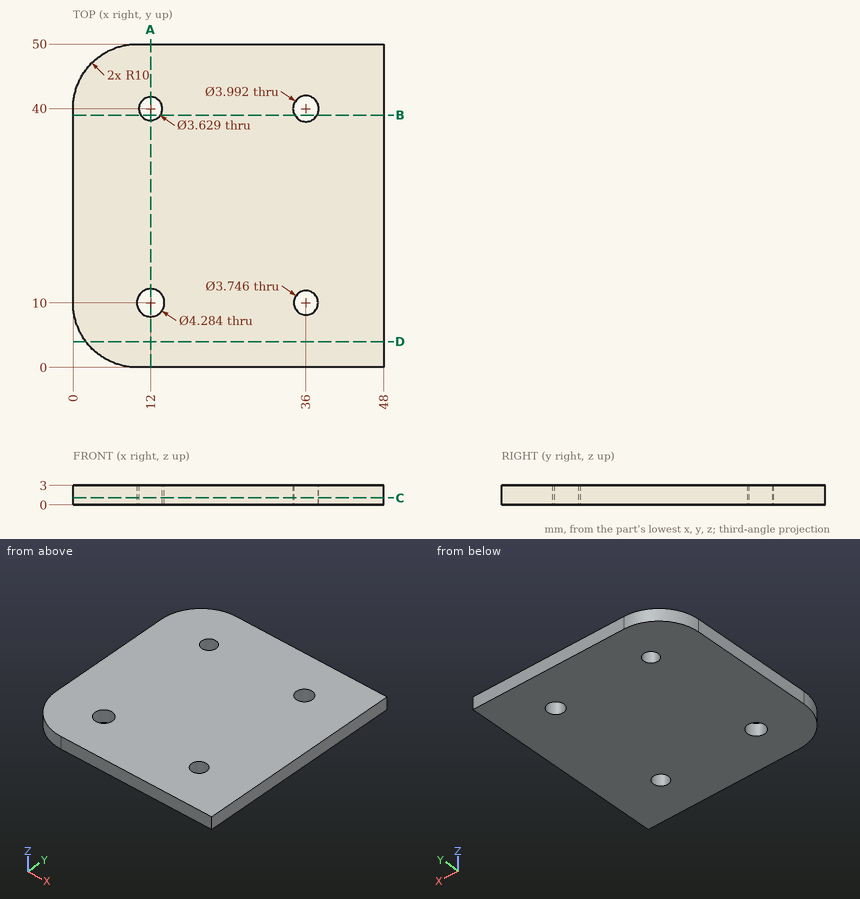
Can you work these out from the drawing? Everything is in mm from the part's minimum corner. Give positions to 0.01 mm unless a question says otherwise; leave off trailing zeros. Order: outer loops, then holes, each group sorted by start corner. A loop starts at its lowest first (then second) coordinate and runs counter-clockwise, first axis right, second up.
1. Suppose I cut it at A-A (x = 12). List the corners of the cut face in (y, z) for me (1 decimal).
2. Suppose I cut it at D-D (y = 4). List the corners of the cut face in (x, z) for me.
3. Suppose I cut it at B-B (y = 39). List the corners of the cut face in (x, z) for me.
4. Suppose I cut it at C-C (z = 1.1). List the corners of the cut face in (x, y) for me (1 decimal), plus the area to 3 significant figures.
5. I need wall thicknesses on L1, parallel to Y at x = 36, z = 1.75 (1 decimal); L2, parallel to Y at x = 36.5, z = 1.15 (1 decimal); L3, parallel to X at y = 39.5, z = 0.8 (1 decimal). Which ranges of each line are inside material? Lowest first, please.
Solved:
1. outline: (0, 0) - (7.9, 0) - (7.9, 3) - (0, 3) - close; (12.1, 0) - (38.2, 0) - (38.2, 3) - (12.1, 3) - close; (41.8, 0) - (50, 0) - (50, 3) - (41.8, 3) - close
2. outline: (2, 0) - (48, 0) - (48, 3) - (2, 3) - close
3. outline: (0, 0) - (10.49, 0) - (10.49, 3) - (0, 3) - close; (13.51, 0) - (34.27, 0) - (34.27, 3) - (13.51, 3) - close; (37.73, 0) - (48, 0) - (48, 3) - (37.73, 3) - close
4. outline: (0, 10) arc R10 ccw to (10, 0) - (48, 0) - (48, 50) - (10, 50) arc R10 ccw to (0, 40) - close; hole circle Ø4.3 at (12, 10); hole circle Ø3.6 at (12, 40); hole circle Ø4 at (36, 40); hole circle Ø3.7 at (36, 10)
4. area: 2,310 mm2
5. L1: y = 0 to 8.1, 11.9 to 38, 42 to 50
5. L2: y = 0 to 8.2, 11.8 to 38.1, 41.9 to 50
5. L3: x = 0 to 10.3, 13.7 to 34.1, 37.9 to 48
